from build123d import *

# Parameters (mm, degrees)
BOSS_EXTRUDE1_DEPTH = 31
SKETCH3_R           = 2.5
BOSS_EXTRUDE2_DEPTH = 11
FILLET1_R           = 1


with BuildPart() as part:
    # Sketch2 → Boss-Extrude1 (new body)
    with BuildSketch(Plane.XY):
        with BuildLine():
            Line((-7.937253933, 9), (7.937253933, 9))
            ThreePointArc((7.937253933, 9), (12, 0), (7.937253933, -9))
            Line((7.937253933, -9), (-7.937253933, -9))
            ThreePointArc((-7.937253933, -9), (-12, 0), (-7.937253933, 9))
        make_face()
    extrude(amount=BOSS_EXTRUDE1_DEPTH)

    # Sketch3 → Boss-Extrude2 (add)
    with BuildSketch(Plane.XY.offset(31)):
        Circle(SKETCH3_R)
    extrude(amount=BOSS_EXTRUDE2_DEPTH)

    # Fillet1
    fillet1_edges = [part.edges().sort_by_distance(p)[0] for p in [
        (0, -9, 31),
        (-12, 0, 31),
        (0, 9, 31),
        (-12, 0, 0),
        (0, -9, 0),
        (12, 0, 0),
        (0, 9, 0),
        (-7.937253933, 9, 15.5),
        (-7.937253933, -9, 15.5),
        (7.937253933, -9, 15.5),
        (7.937253933, 9, 15.5),
        (12, 0, 31),
    ]]
    fillet(fillet1_edges, radius=FILLET1_R)


solid = part.part
Work out the finished part from the listing and answer in its coordinate system (mm). A direction names the side the tool comes from. Coordinates: 2 decimals unless noted, no trailing zeros. Loops run counter-clockwise (first coordinate to the right, second up) from the corner with the lowest first, then second, coordinate; pieces in that order, holes last. Notation, with made-up numbers: (-23, 47) -> (16, 47) arc R17 cw to (16, 55) -> close; hole circle Ø10 at (15, 42.25). An arc over 180 degrees is marked (long way). Answer as CSV lines item,"result".
1) Flat-ended cylindrical pins translate along their axes: pin 1 (2 mm diameter, centred on y = -6.5, z = 13.5, fed in from +X); pin 2 (2 mm diameter, centred on y = 4.5, z = 11, fed in from -X). Find the tip coordinate at first contact, or state that the pin passes through.
A:
pin 1,"stops at x = 10.67"
pin 2,"stops at x = -11.48"
2) The part is cut by section D-D (x = 5.75). Give the vertices of the cut face in (y, z).
A:
outline,"(-9, 1) arc R1 ccw to (-8, 0) -> (8, 0) arc R1 ccw to (9, 1) -> (9, 30) arc R1 ccw to (8, 31) -> (-8, 31) arc R1 ccw to (-9, 30) -> close"
3) Straight lines are drawn through the part: probe 1 along Z at (x, y) = (-9.25, 0.75); probe 2 along Y at (x, z) = (-0.75, 33.5); probe 3 along X at (y, z) = (-5.75, 25). For each, find the intervals that lie inside material, in ascending order.
A:
probe 1,"z = 0 to 31"
probe 2,"y = -2.38 to 2.38"
probe 3,"x = -10.53 to 10.53"
4) The part is cut by section C-C (y = 0). Give the vertices of the cut face in (x, z), and give its area (3 significant figures).
A:
outline,"(-12, 1) arc R1 ccw to (-11, 0) -> (11, 0) arc R1 ccw to (12, 1) -> (12, 30) arc R1 ccw to (11, 31) -> (2.5, 31) -> (2.5, 42) -> (-2.5, 42) -> (-2.5, 31) -> (-11, 31) arc R1 ccw to (-12, 30) -> close"
area,"798 mm²"
5) For faces 4 (the face through (-0.106, -8.699, 0.285)), 5 (the face through (-0.54, -2.44, 36.42)), determine the directions among +Z, -Z, +X, -X, +Y, -Y from which every point of the face is accessible in a straight line to the end or side of a thin tool.
A:
face 4,"-Z, +X, -X, -Y"
face 5,"+Z"
6) For a pull along Z with two mould halves and no side action, classify faces 1 (the face through (0, 0, 0)), 2 (the face through (3, 0, 31)), 3 (the face through (0, 9, 15)) as released by +Z, released by -Z, zero draft, split by the parting line, or undercut.
A:
face 1,"released by -Z"
face 2,"released by +Z"
face 3,"zero draft"
7) The part is cut by section B-B (z = 5). Give the vertices of the cut face in (x, y), and give its area (3 significant figures).
A:
outline,"(-8.24, -8.73) arc R1 ccw to (-7.55, -9) -> (7.55, -9) arc R1 ccw to (8.24, -8.73) arc R12 ccw to (8.24, 8.73) arc R1 ccw to (7.55, 9) -> (-7.55, 9) arc R1 ccw to (-8.24, 8.73) arc R12 ccw to start"
area,"387 mm²"
8) The part is cut by section A-A (x = 0). Give the vertices of the cut face in (y, z), and give its area (3 significant figures).
A:
outline,"(-9, 1) arc R1 ccw to (-8, 0) -> (8, 0) arc R1 ccw to (9, 1) -> (9, 30) arc R1 ccw to (8, 31) -> (2.5, 31) -> (2.5, 42) -> (-2.5, 42) -> (-2.5, 31) -> (-8, 31) arc R1 ccw to (-9, 30) -> close"
area,"612 mm²"
